from build123d import *

# Parameters (mm, degrees)
F0_W      = 1320.8
F0_H      = 457.2
F1_DEPTH  = 152.4
F2_R      = 50.8
F2_R_2    = 12.7
F3_DEPTH  = 25.4
F6_DEPTH  = 304.8
F7_T      = 3.175
F8_W      = 152.4
F8_H      = 44.45
F9_DEPTH  = 6.35
F11_R     = 9.525
F12_DEPTH = 12.7
F10_R     = 12.7
F13_DEPTH = 12.7


with BuildPart() as f1:
    # F0 (on Front) → F1 (new body, symmetric)
    with BuildSketch(Plane.XZ):
        Rectangle(F0_W, F0_H)
    extrude(amount=F1_DEPTH, both=True)

    # F2 (on face) → F3 (cut, symmetric)
    with BuildSketch(Plane.XY.offset(228.6)):
        with Locations((482.6, 0)):
            Circle(F2_R)
        Circle(F2_R_2)
        with Locations((-609.6, -101.6)):
            Circle(F2_R_2)
    extrude(amount=F3_DEPTH, both=True, mode=Mode.SUBTRACT)

    # F5 (on face) → F6 (cut, through all)
    with BuildSketch(Plane.XZ.offset(152.4)):
        Polygon((-559.0197953224, -233.4262882042), (-660.6197953224, -126.7462882042), (-660.6197953224, -233.4262882042), align=None)
        Polygon((660.6197953224, -126.7462882042), (559.0197953224, -233.4262882042), (660.6197953224, -233.4262882042), align=None)
    extrude(amount=-F6_DEPTH, mode=Mode.SUBTRACT)

    # F7 (hollow, outwards: the wall grows on the outside; the body as it was is the cavity)
    f7_inside = f1.part
    offset(amount=F7_T, kind=Kind.INTERSECTION)
    add(f7_inside, mode=Mode.SUBTRACT)

    # F8 (on face) → F9 (join)
    with BuildSketch(Plane(origin=(0, 0, -231.775), x_dir=(1, 0, 0), z_dir=(0, 0, -1))):
        with Locations((583.1482922554, -57.15)):
            Rectangle(F8_W, F8_H)
        with Locations((583.1482922554, 57.15)):
            Rectangle(F8_W, F8_H)
    extrude(amount=F9_DEPTH)

    # F11 (on face) → F12 (cut, symmetric)
    with BuildSketch(Plane.XY.offset(231.775)):
        with Locations((-325.7964868545, 0)):
            Circle(F11_R)
    extrude(amount=F12_DEPTH, both=True, mode=Mode.SUBTRACT)

    # F10 (on face) → F13 (cut, symmetric)
    with BuildSketch(Plane(origin=(0, 0, -231.775), x_dir=(1, 0, 0), z_dir=(0, 0, -1))):
        Circle(F10_R)
    extrude(amount=F13_DEPTH, both=True, mode=Mode.SUBTRACT)


solid = f1.part
The listing builds one solid part. Answer for the finished solid, in the listing's coordinates (mm). A direction names the side the tool comes from. Give positions to 0.01 mm unless a question says otherwise; leave off trailing zeros. Order: outer loops, then holes, each group sorted by start corner. A loop starts at its lowest first (then second) coordinate and runs counter-clockwise, first axis right, second up. Notation, with made-up numbers: (19, -22) - (52, -22) arc R25 cw to (52, -8) - close; hole circle Ø7 at (-3.75, -7). An arc over 180 degrees is marked (long way). Answer as CSV lines item,"result".
Q1. Each of these flat-tipped pins is pushed along its axis until it touches: pin 1 Ø1.9 at (y, z) = (-47.5, -235) entering from +X; pin 2 Ø6 at (x, y) = (-336.5, -83) entering from -Z (3 decimals); pin 3 Ø3 at (y, z) = (49.5, -234.5) entering from -X. Where does it stop, or does it pass through?
Answer key:
pin 1,"stops at x = 659.35"
pin 2,"stops at z = -231.775"
pin 3,"stops at x = 506.95"
Q2. Determine the mould class of faces 1 (the face through (-2.75, 12.4, -230.21)), 2 (the face through (-9, -155.575, 3)), 3 (the face through (-9, -37, 231.775)) for opening direction Y: pulls with the +Y half, pulls with the -Y half, needs draft (parallel to the pull), parting line crosses it, or undercut.
Answer key:
face 1,"undercut"
face 2,"pulls with the -Y half"
face 3,"needs draft"
Q3. Which of the six approach directions +Z, -Z, +X, -X, +Y, -Y give full straight-line access (tool end or side, diameter ignored) to faces 4 (the face through (-2.75, -12.4, 216.08)), 5 (the face through (504.58, -42.25, 219.25)), 6 (the face through (612, -57, -231.775))?
Answer key:
face 4,"none"
face 5,"+Z"
face 6,"+X, +Y, -Y"
Q4. A cutting plane is placed at A-A, the plane x = -296. Determine the outline of the cut face in (y, z) (3 decimals).
Answer key:
outline,"(-155.575, -231.775) - (155.575, -231.775) - (155.575, 231.775) - (-155.575, 231.775) - close; hole (-152.4, -228.6) - (152.4, -228.6) - (152.4, 228.6) - (-152.4, 228.6) - close"
Q5. A cutting plane is placed at D-D, the plane x = 482.6. Determine the outline of the cut face in (y, z) (3 decimals).
Answer key:
outline,"(-155.575, -231.775) - (155.575, -231.775) - (155.575, 231.775) - (47.625, 231.775) - (47.625, 206.375) - (-47.625, 206.375) - (-47.625, 231.775) - (-155.575, 231.775) - close; hole (-152.4, -228.6) - (152.4, -228.6) - (152.4, 228.6) - (50.8, 228.6) - (50.8, 203.2) - (-50.8, 203.2) - (-50.8, 228.6) - (-152.4, 228.6) - close"
Q6. A cutting plane is placed at B-B, the plane z = 137.5. Determine the outline of the cut face in (x, y) (3 decimals).
Answer key:
outline,"(-663.575, -155.575) - (663.575, -155.575) - (663.575, 155.575) - (-663.575, 155.575) - close; hole (-660.4, -152.4) - (660.4, -152.4) - (660.4, 152.4) - (-660.4, 152.4) - close"
Q7. Straight lines are drawn through the part: L1, parallel to Y at x = 482, z = 224 (3 decimals); L2, parallel to X at y = 61, z = 20 (3 decimals); L3, parallel to Z at x = -348.5, y = 13 (3 decimals). For each, find the intervals that lie inside material, in ascending order.
Answer key:
L1,"y = -155.575 to -152.4, -50.796 to -47.621, 47.621 to 50.796, 152.4 to 155.575"
L2,"x = -663.575 to -660.4, 660.4 to 663.575"
L3,"z = -231.775 to -228.6, 228.6 to 231.775"
Q8. A cutting plane is placed at C-C, the plane y = 108. Determine the outline of the cut face in (x, z) (3 decimals).
Answer key:
outline,"(-663.575, -128.247) - (-564.977, -231.775) - (564.977, -231.775) - (663.575, -128.247) - (663.575, 231.775) - (-663.575, 231.775) - close; hole (-660.4, -126.977) - (-563.616, -228.6) - (563.616, -228.6) - (660.4, -126.977) - (660.4, 228.6) - (-660.4, 228.6) - close"
